Print and shaded views of the part. All mm, measured from the part's lowest x, y and z. A direction names the side the tool comes from. Round coordinates to 2 decimals unless told otherwise and drop trailing zeros. Loops run counter-clockwise (first coordinate to the right, second up) from the corner with the lowest first, then second, coordinate; pieces in that order, holes last. Notation, with made-up numbers: (37.5, 33.25) - (92.5, 33.25) arc R19 ccw to (92.5, 63.25) - close; hole circle Ø2 at (22, 30.5). An arc over 180 degrees is marked (long way). Answer as a JSON object with one key per item and string values.
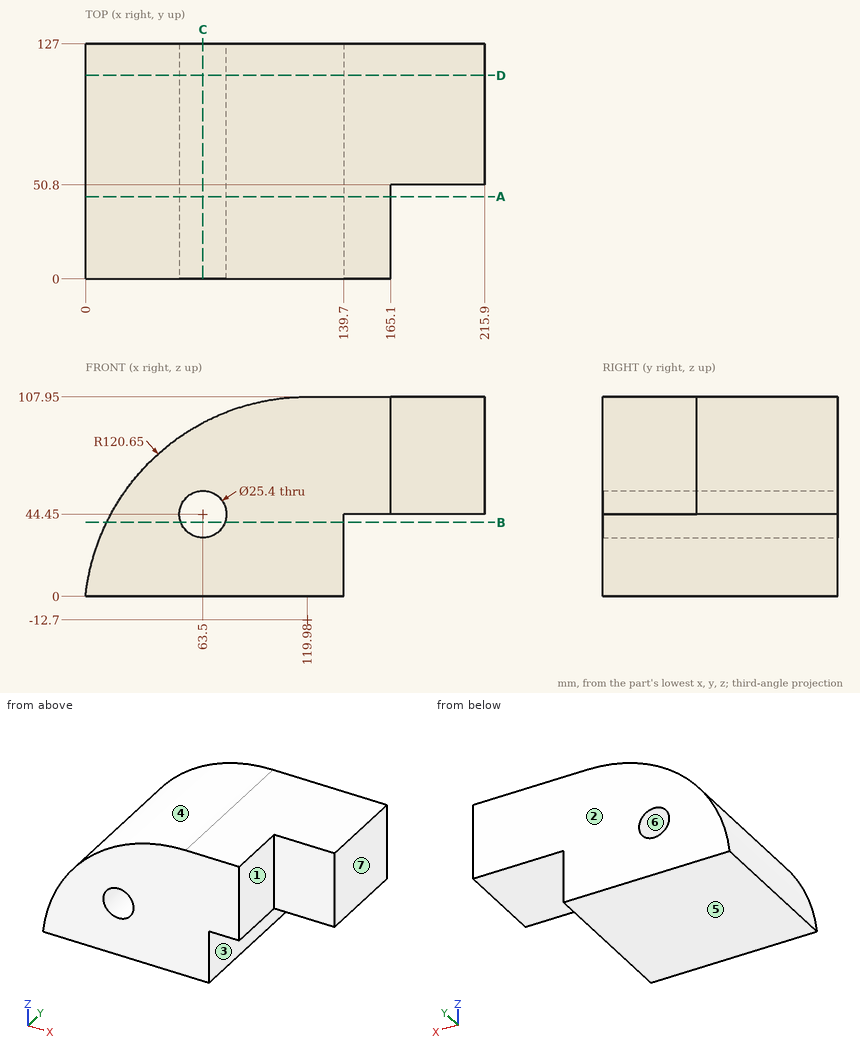
1) Slice it at A-A on y = 44.5. List the corners of the cut face in (x, z).
Values follow:
{"outline": "(0, 0) - (139.7, 0) - (139.7, 44.45) - (165.1, 44.45) - (165.1, 107.95) - (119.98, 107.95) arc R120.65 ccw to start; hole circle Ø25.4 at (63.5, 44.45)"}
2) Probe probe 1 along Z at (x, y) = (63.5, 35); probe 2 along Z at (x, y) = (63, 89); probe 3 along Z at (x, y) = (155, 68). List the from-to ranges inside material, lowest first.
Values follow:
{"probe 1": "0 to 31.75, 57.15 to 93.91", "probe 2": "0 to 31.76, 57.14 to 93.65", "probe 3": "44.45 to 107.95"}
3) Tool access for the marked faces 1, 2 and 3: list every direction of +Z, -Z, +X, -X, +Y, -Y with a clear straight run to the whole face (end or side of a thin tool).
Values follow:
{"face 1": "+Z, -Z, +X, -Y", "face 2": "+Z, -Z, +X, -X, +Y", "face 3": "-Z, +X, +Y, -Y"}
4) Two-plate mould, pull along Z, no slides. Class the marked faces 4, 5, 6 and 7: pulls with the +Z half, pulls with the -Z half, needs draft (parallel to the pull), parting line crosses it, or undercut.
Values follow:
{"face 4": "pulls with the +Z half", "face 5": "pulls with the -Z half", "face 6": "undercut", "face 7": "needs draft"}
5) Slice it at D-D on y = 110. List the corners of the cut face in (x, z), then the cut area to 3 significant figures.
Values follow:
{"outline": "(0, 0) - (139.7, 0) - (139.7, 44.45) - (215.9, 44.45) - (215.9, 107.95) - (119.98, 107.95) arc R120.65 ccw to start; hole circle Ø25.4 at (63.5, 44.45)", "area": "16,400 mm²"}
6) Slice it at B-B on z = 40. List the corners of the cut face in (x, y) (1 decimal).
Values follow:
{"outline": "(11.4, 0) - (51.6, 0) - (51.6, 127) - (11.4, 127) - close; (75.4, 0) - (139.7, 0) - (139.7, 127) - (75.4, 127) - close"}
7) Drop flat-ended pins along their axis: P1, Ø23, axis at x = 178, y = 89, coming from the -Z side; P2, Ø10, axis at y = 61.5, z = 53, coming from the -X side; P3, Ø22, axis at y = 87, z = 29, coming from the +X side; P4, Ø2, axis at x = 64, z = 54.5, coming from the +Y side. Give the stop position or say it passes through.
Values follow:
{"P1": "z = 44.45", "P2": "x = 15.71", "P3": "x = 139.7", "P4": "through"}
8) Slice it at C-C on x = 63.5. List the corners of the cut face in (y, z).
Values follow:
{"outline": "(0, 0) - (127, 0) - (127, 31.75) - (0, 31.75) - close; (0, 57.15) - (127, 57.15) - (127, 93.91) - (0, 93.91) - close"}
